from build123d import *

# Parameters (mm, degrees)
CROQUIS1_W                    = 165
CROQUIS1_H                    = 3.175
BRIDA_BASE1_DEPTH             = 25.4
BRIDA_DE_ARISTA1_DEPTH        = 25.4
BRIDA_DE_ARISTA1_BEND_DEPTH   = 25.4
BRIDA_DE_ARISTA2_DEPTH        = 25.4
BRIDA_DE_ARISTA2_BEND_DEPTH   = 25.4
TALADRO_DE_MARGEN_PARA_3_81_D = 10.0838


# Sheet-metal steps are written as plain solids
with BuildPart() as part:
    # Croquis1 → Brida base1 (new body)
    with BuildSketch(Plane.XY):
        with Locations((6.420112782, -1.5875)):
            Rectangle(CROQUIS1_W, CROQUIS1_H)
    extrude(amount=BRIDA_BASE1_DEPTH)

    # Brida de arista1 section (across the edge) → Brida de arista1 (add)
    with BuildSketch(Plane(origin=(89.656712782, -3.175, 0), x_dir=(-1, 0, 0), z_dir=(0, 0, 1))):
        with BuildLine():
            Line((-3.175, 0.7366), (-3.175, 81.825))
            Line((-3.175, 81.825), (0, 81.825))
            Line((0, 81.825), (0, 0.7366))
            ThreePointArc((0, 0.7366), (0.215745145, 0.215745145), (0.7366, 0))
            Line((0.7366, 0), (0.7366, -3.175))
            ThreePointArc((0.7366, -3.175), (-2.029318885, -2.029318885), (-3.175, 0.7366))
        make_face()
    extrude(amount=BRIDA_DE_ARISTA1_DEPTH)

    # Brida de arista1 section 2 (across the edge) → Brida de arista1 bend (add)
    with BuildSketch(Plane(origin=(-76.816487218, -3.175, 25.4), x_dir=(1, 0, 0), z_dir=(0, 0, -1))):
        with BuildLine():
            Line((-3.175, 0.7366), (-3.175, 81.825))
            Line((-3.175, 81.825), (0, 81.825))
            Line((0, 81.825), (0, 0.7366))
            ThreePointArc((0, 0.7366), (0.215745145, 0.215745145), (0.7366, 0))
            Line((0.7366, 0), (0.7366, -3.175))
            ThreePointArc((0.7366, -3.175), (-2.029318885, -2.029318885), (-3.175, 0.7366))
        make_face()
    extrude(amount=BRIDA_DE_ARISTA1_BEND_DEPTH)

    # Brida de arista2 section (across the edge) → Brida de arista2 (add)
    with BuildSketch(Plane(origin=(92.831712782, -85.7366, 25.4), x_dir=(0, 1, 0), z_dir=(0, 0, -1))):
        with BuildLine():
            Line((-3.175, 0.7366), (-3.175, 24.825))
            Line((-3.175, 24.825), (0, 24.825))
            Line((0, 24.825), (0, 0.7366))
            ThreePointArc((0, 0.7366), (0.215745145, 0.215745145), (0.7366, 0))
            Line((0.7366, 0), (0.7366, -3.175))
            ThreePointArc((0.7366, -3.175), (-2.029318885, -2.029318885), (-3.175, 0.7366))
        make_face()
    extrude(amount=BRIDA_DE_ARISTA2_DEPTH)

    # Brida de arista2 section 2 (across the edge) → Brida de arista2 bend (add)
    with BuildSketch(Plane(origin=(-79.991487218, -85.7366, 0), x_dir=(0, 1, 0), z_dir=(0, 0, 1))):
        with BuildLine():
            Line((-3.175, 0.7366), (-3.175, 24.825))
            Line((-3.175, 24.825), (0, 24.825))
            Line((0, 24.825), (0, 0.7366))
            ThreePointArc((0, 0.7366), (0.215745145, 0.215745145), (0.7366, 0))
            Line((0.7366, 0), (0.7366, -3.175))
            ThreePointArc((0.7366, -3.175), (-2.029318885, -2.029318885), (-3.175, 0.7366))
        make_face()
    extrude(amount=BRIDA_DE_ARISTA2_BEND_DEPTH)

    # Taladro de margen para 3/81 (through all)
    with Locations(Plane(origin=(0, -88.9116, 0), x_dir=(-1, 0, 0), z_dir=(0, -1, 0))):
        with Locations((93.586487218, -12.7), (-106.413512782, -12.7)):
            Hole(TALADRO_DE_MARGEN_PARA_3_81_D / 2)


solid = part.part
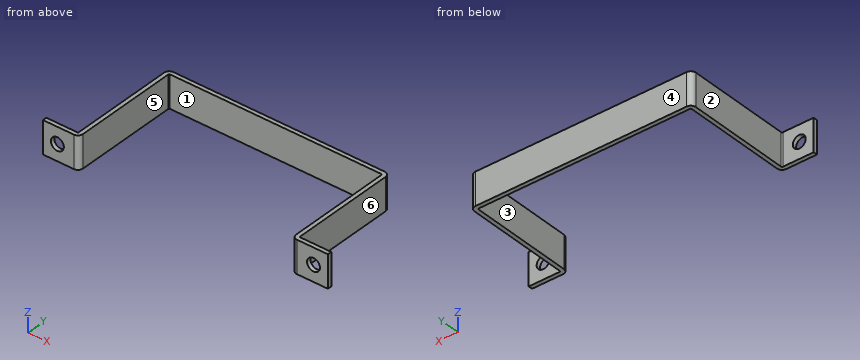
Read the model definition and answer for the solid it produces. Units are mm, in the model's axes. Face numbers are marked on the shaded views. A direction names the side the tool comes from. Round coordinates to 2 decimals unless told otherwise and drop trailing zeros. Write each loop counter-clockwise with the first axis right and the second up, starting at its lowest first coordinate (ties: lowest second). Pieces come first, ordered by that corner, then holes.
1. The part is cut by section B-B, the plane z = 12.7. Determine the outline of the cut face in (x, y) (3 decimals), then the cut area to 3 significant figures.
2. Given pin 1 Ø12 at (x, z) = (104, 16.5) entering from +Y; pin 2 Ø12.5 at (x, z) = (38, 17.5) entering from -Y (3 decimals); pin 3 Ø6 at (y, z) = (-27, 22.5) entering from -X; pin 4 Ø1 at (x, y) = (-75, -59) entering from +Z, each flat-ended and moving along its own axis, determine where each tip first touches the part or whether it passes through.
3. Determine the mould class of the marked faces 1, 2, 3 and 4 for opening direction X: pulls with the +X half, pulls with the -X half, needs draft (parallel to the pull), parting line crosses it, or undercut.
4. The part is cut by section C-C, the plane z = 2. Determine the outline of the cut face in (x, y) (3 decimals), then the cut area to 3 significant figures.
5. Straight lines are drawn through the part: L1, parallel to X at y = -40, z = 16.25; L2, parallel to Y at x = 88, z = 21.5 (3 decimals); L3, parallel to Y at x = 89.5, z = 2. For each, find the intervals that lie inside material, in ascending order.
6. Which of the six approach directions +Z, -Z, +X, -X, +Y, -Y give full straight-line access (tool end or side, diameter ignored) to the marked faces 5 and 6?
7. The part is cut by section A-A, the plane y = -59.5. Determine the outline of the cut face in (x, z).
8. The part is cut by section D-D, the plane x = 7.5. Determine the outline of the cut face in (y, z) (3 decimals), then the cut area to 3 significant figures.
Values:
1. outline: (-104.816, -88.912) - (-98.628, -88.912) - (-98.628, -85.737) - (-104.816, -85.737) - close; (-88.545, -88.912) - (-80.728, -88.912) arc R3.912 ccw to (-76.816, -85) - (-76.816, -3.912) arc R0.737 cw to (-76.08, -3.175) - (88.92, -3.175) arc R0.737 cw to (89.657, -3.912) - (89.657, -85) arc R3.912 ccw to (93.568, -88.912) - (101.372, -88.912) - (101.372, -85.737) - (93.568, -85.737) arc R0.737 cw to (92.832, -85) - (92.832, -3.912) arc R3.912 ccw to (88.92, 0) - (-76.08, 0) arc R3.912 ccw to (-79.991, -3.912) - (-79.991, -85) arc R0.737 cw to (-80.728, -85.737) - (-88.545, -85.737) - close; (111.455, -88.912) - (117.657, -88.912) - (117.657, -85.737) - (111.455, -85.737) - close
1. area: 1,170 mm2
2. pin 1: stops at y = -85.74
2. pin 2: stops at y = -3.175
2. pin 3: stops at x = -79.99
2. pin 4: passes through
3. face 1: undercut
3. face 2: pulls with the -X half
3. face 3: undercut
3. face 4: needs draft
4. outline: (-104.816, -88.912) - (-80.728, -88.912) arc R3.912 ccw to (-76.816, -85) - (-76.816, -3.912) arc R0.737 cw to (-76.08, -3.175) - (88.92, -3.175) arc R0.737 cw to (89.657, -3.912) - (89.657, -85) arc R3.912 ccw to (93.568, -88.912) - (117.657, -88.912) - (117.657, -85.737) - (93.568, -85.737) arc R0.737 cw to (92.832, -85) - (92.832, -3.912) arc R3.912 ccw to (88.92, 0) - (-76.08, 0) arc R3.912 ccw to (-79.991, -3.912) - (-79.991, -85) arc R0.737 cw to (-80.728, -85.737) - (-104.816, -85.737) - close
4. area: 1,240 mm2
5. L1: x = -79.99 to -76.82, 89.66 to 92.83
5. L2: y = -3.175 to 0
5. L3: y = -3.46 to -0.04
6. face 5: +Z, -Z, -Y
6. face 6: +Z, -Z, +X, +Y
7. outline: (-79.99, 0) - (-76.82, 0) - (-76.82, 25.4) - (-79.99, 25.4) - close; (89.66, 0) - (92.83, 0) - (92.83, 25.4) - (89.66, 25.4) - close
8. outline: (-3.175, 0) - (0, 0) - (0, 25.4) - (-3.175, 25.4) - close
8. area: 80.6 mm2
